from build123d import *

# Parameters (mm, degrees)
BOSS_EXTRUDE1_DEPTH = 40
BOSS_EXTRUDE2_DEPTH = 16


with BuildPart() as part:
    # Sketch1 → Boss-Extrude1 (new body)
    with BuildSketch(Plane.XY):
        Polygon((0, 0), (0, 35), (-18, 35), (-18, 13), (-40, 13), (-40, 0), align=None)
    extrude(amount=-BOSS_EXTRUDE1_DEPTH)

    # Sketch2 → Boss-Extrude2 (add)
    with BuildSketch(Plane(origin=(0, 0, -40), x_dir=(-1, 0, 0), z_dir=(0, 0, -1))):
        Polygon((18, 13), (18, 25), (54.657821702, 25), (54.657821702, 0), (40, 0), (40, 13), align=None)
    extrude(amount=-BOSS_EXTRUDE2_DEPTH)


solid = part.part
The model under review builds one solid part; all positions refer to its coordinate system, in mm. A direction names the side the tool comes from. Round coordinates to 2 decimals unless told otherwise and drop trailing zeros. Loops run counter-clockwise (first coordinate to the right, second up) from the corner with the lowest first, then second, coordinate; pieces in that order, holes last. Notation, with made-up numbers: M 36,-7.5 L 45,-7.5 A7 cw 45,-3.5 Z; hole C 18.25,70.5 d11. An arc over 180 degrees is marked long. Answer as CSV lines item,"result". Start each with the question number.
Item 1: Consider section C-C (x = -42). Write out the cut boundary in (y, z).
Item 2: Wall thickness on line 1 (Z direction, x = -44, y = 4.5); line 2 (X direction, y = 30, z = -22.5); line 3 (Y direction, x = -25.5, z = -23.5): over which ranges is each line inside the solid? List them lowest first. Write a range as [from, to].
Item 3: Consider section A-A (y = 14). Write out the cut boundary in (x, z), then the cut area to 3 significant figures.
Item 4: Consider section B-B (x = -26). Write out the cut boundary in (y, z).
Item 5: For faces 1 (the face through (-29, 13, -12)), 2 (the face through (-40, 7, -12)), 3 (the face through (-36, 25, -32)), list the 3-axis set-ups (+Z, -Z, +X, -X, +Y, -Y) from which the entire face can be reached by the end or side of a thin tool; tool diameter is ignored.
Item 6: Insertion check: P1, Ø14.5, axis at y = 6.5, z = -7.5, coming from the -X side; P2, Ø2, axis at x = -34.5, z = -13, coming from the +Y side; P3, Ø17.5, axis at y = 23.5, z = -10, coming from the -X side. Each pin has a flat end and moves straight along its axis. Give the tip position at first contact, or say it passes through.
Answer:
1,outline,"M 0,-40 L 25,-40 L 25,-24 L 0,-24 Z"
2,line 1,"z = [-40, -24]"
2,line 2,"x = [-18, 0]"
2,line 3,"y = [0, 13]"
3,outline,"M -54.66,-40 L 0,-40 L 0,0 L -18,0 L -18,-24 L -54.66,-24 Z"
3,area,"1,310 mm^2"
4,outline,"M 0,-40 L 25,-40 L 25,-24 L 13,-24 L 13,0 L 0,0 Z"
5,face 1,"+Z, -X, +Y"
5,face 2,"+Z, -X, +Y, -Y"
5,face 3,"+Z, -Z, -X, +Y"
6,P1,"stops at x = -40"
6,P2,"stops at y = 13"
6,P3,"stops at x = -18"
